Verification items for the finished model (mm, model axes). A direction names the side the tool comes from. Give positions to 0.01 mm unless a question says otherwise; leave off trailing zeros. Loops run counter-clockwise (first coordinate to the right, second up) from the corner with the lowest first, then second, coordinate; pieces in that order, holes last. Notation, with made-up numbers: (19.5, 7.5) - (46.5, 7.5) arc R19 ccw to (46.5, 23.5) - close; hole circle Ø8 at (39.5, 42.25). An arc over 180 degrees is marked (long way). One line per item, written item: value. Start each with the question number.
1. Access from +Z, -Z, +X, -X, +Y, -Y to the whole of each face (thin tool, end or side, straight path). Record for faces 1 (the flat face through (25, -8, 0)), 2 (the flat face through (25, 0, 19)), 3 (the flat face through (38.1, -26, 40)), 4 (the flat face through (12.7, -26, 40)).
2. Sectioned sample at A-A (x = 25.4). Record the cut outline in (y, z) (3 decimals), plus the area to 3 significant figures.
3. Gauge pin test, flat ends, axial feed: pin 1 (2 mm diameter, centred on y = -15, z = -27, fed in from -X); pin 2 (6 mm diameter, centred on y = -26, z = -35.5, fed in from +X); pin 3 (1 mm diameter, centred on x = 22.5, z = 52.5, fed in from -Y). Record the tip position at first contact, or that the pin passes through.
4. Sectioned sample at C-C (y = -2.5). Record the cut outline in (x, z), plus the area to 3 significant figures.
5. Mould release check, pull along Y, two halves, no side actions. Record for faces 5 (the cylindrical face through (25.58, -20.28, 58.83)), 6 (the flat face through (50.8, -26, 6)), 7 (the cylindrical face through (16.04, -33.983, -38.246)): pulls with the +Y half, pulls with the -Y half, needs draft (parallel to the pull), parting line crosses it, or undercut.
6. Scan lines: L1, parallel to Z at x = 31, y = -25; L2, parallel to Y at x = 26, z = 50; L3, parallel to Z at x = 46, y = -24. Record each from-to range of solid material in increasing order. Write a range as [from, to].
7. Sectioned sample at D-D (x = 5). Record the cut outline in (y, z), plus the area to 3 significant figures.
8. Sectioned sample at B-B (y = -25.4). Record the cut outline in (x, z) (3 decimals).
from build123d import *

# Parameters (mm, degrees)
F0_W      = 50.8
F0_H      = 50.8
F1_DEPTH  = 12.7
F3_R      = 12.7
F4_DEPTH  = 76.2
F5_W      = 50.8
F5_H      = 38.1
F6_DEPTH  = 38.1
F7_DEPTH  = 12.7
F8_R      = 9.525
F9_DEPTH  = 38.101
F10_R     = 3.81
F11_SIZE2 = 2.54
F11_SIZE  = 2.54


with BuildPart() as f1:
    # F0 (on Top) → F1 (new body)
    with BuildSketch(Plane.XY):
        with Locations((25.4, -25.4)):
            Rectangle(F0_W, F0_H)
    extrude(amount=F1_DEPTH)

    # F3 (on face) → F4 (join)
    with BuildSketch(Plane(origin=(0, 0, 0), x_dir=(1, 0, 0), z_dir=(0, 0, -1))):
        with Locations((25.4, 25.4)):
            Circle(F3_R)
    extrude(amount=F4_DEPTH)

    # F5 (on Right) → F6 (join)
    with BuildSketch(Plane.YZ):
        with BuildLine():
            ThreePointArc((0, 50.8), (-25.4, 76.2), (-50.8, 50.8))
            Line((-50.8, 50.8), (0, 50.8))
        make_face()
        with Locations((-25.4, 31.75)):
            Rectangle(F5_W, F5_H)
    extrude(amount=F6_DEPTH)

    # F5 (on Right) → F7 (cut)
    with BuildSketch(Plane.YZ):
        with BuildLine():
            ThreePointArc((0, 50.8), (-25.4, 76.2), (-50.8, 50.8))
            Line((-50.8, 50.8), (0, 50.8))
        make_face()
        with Locations((-25.4, 31.75)):
            Rectangle(F5_W, F5_H)
    extrude(amount=F7_DEPTH, mode=Mode.SUBTRACT)

    # F8 (on face) → F9 (cut, through all)
    with BuildSketch(Plane.YZ.offset(38.1)):
        with Locations((-25.4, 50.8)):
            Circle(F8_R)
    extrude(amount=-F9_DEPTH, mode=Mode.SUBTRACT)

    # F10
    f10_edges = [f1.edges().sort_by_distance(p)[0] for p in [
        (38.1, -25.4, 12.7),
        (12.7, -25.4, 12.7),
        (12.7, -25.4, 0),
    ]]
    fillet(f10_edges, radius=F10_R)

    # F11
    f11_edges = [f1.edges().sort_by_distance(p)[0] for p in [
        (12.7, -25.4, -76.2),
    ]]
    chamfer(f11_edges, length=F11_SIZE, length2=F11_SIZE2)


solid = f1.part
Results are:
1. face 1: -Z
1. face 2: +Z, -Z, +X, -X, +Y
1. face 3: +Z, +X, +Y, -Y
1. face 4: +Z, -X, +Y, -Y
2. outline: (-50.8, 0) - (-41.91, 0) arc R3.81 cw to (-38.1, -3.81) - (-38.1, -73.66) - (-35.56, -76.2) - (-15.24, -76.2) - (-12.7, -73.66) - (-12.7, -3.81) arc R3.81 cw to (-8.89, 0) - (0, 0) - (0, 50.8) arc R25.4 ccw to (-50.8, 50.8) - close; hole circle Ø19.05 at (-25.4, 50.8)
2. area: 5,240 mm^2
3. pin 1: stops at x = 16.86
3. pin 2: stops at x = 38.1
3. pin 3: stops at y = -50.77
4. outline: (0, 0) - (50.8, 0) - (50.8, 12.7) - (41.91, 12.7) arc R3.81 cw to (38.1, 16.51) - (38.1, 61.79) - (12.7, 61.79) - (12.7, 16.51) arc R3.81 cw to (8.89, 12.7) - (0, 12.7) - close
4. area: 1,900 mm^2
5. face 5: undercut
5. face 6: needs draft
5. face 7: parting line crosses it
6. L1: z = [-76.2, 41.28], [60.32, 76.2]
6. L2: y = [-50.8, -34.89], [-15.91, 0]
6. L3: z = [0, 12.7]
7. outline: (-50.8, 0) - (0, 0) - (0, 12.7) - (-50.8, 12.7) - close
7. area: 645 mm^2
8. outline: (0, 0) - (8.89, 0) arc R3.81 cw to (12.7, -3.81) - (12.7, -73.66) - (15.24, -76.2) - (35.56, -76.2) - (38.1, -73.66) - (38.1, -3.81) arc R3.81 cw to (41.91, 0) - (50.8, 0) - (50.8, 12.7) - (41.91, 12.7) arc R3.81 cw to (38.1, 16.51) - (38.1, 41.275) - (12.7, 41.275) - (12.7, 16.51) arc R3.81 cw to (8.89, 12.7) - (0, 12.7) - close; (12.7, 60.325) - (38.1, 60.325) - (38.1, 76.2) - (12.7, 76.2) - close
